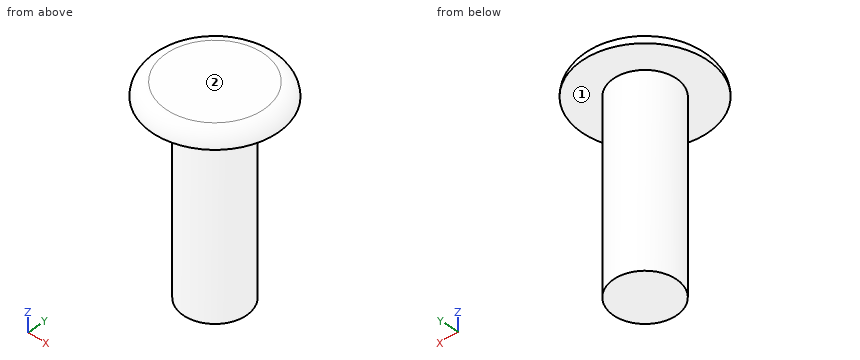
Autodesk Inventor part; units mm, degrees
ref_plane "YZ Plane" through (0, 0, 0) normal (1, 0, 0) x (0, 1, 0)
ref_plane "XZ Plane" through (0, 0, 0) normal (0, 1, 0) x (-1, 0, 0)
ref_plane "XY Plane" through (0, 0, 0) normal (0, 0, 1) x (1, 0, 0)
sketch "スケッチ1" plane through (0, 0, 0) normal (0, 0, 1) x (1, 0, 0)
  circle A0 centre (0, 0) radius 4
  dimension "d0" = 8
extrude "押し出し1" add sketch "スケッチ1" along normal blind 0.9
sketch "スケッチ2" plane through (0, 0, 0) normal (0, 0, -1) x (-1, 0, 0)
  circle A0 centre (0, 0) radius 2
  dimension "d3" = 4
extrude "押し出し2" add sketch "スケッチ2" along normal blind 12
thread "ねじ1"
fillet "フィレット1" radius 0.9 1 edges at (-4, 0, 0.9)
properties part number "ネジ低頭m4.12" material "鋼、高強度、低合金"
Model file for the job. Use its own axes, mm. Face numbers are marked on the shaded views. A direction names the side the tool comes from. Coordinates: 2 decimals unless noted, no trailing zeros. Loops run counter-clockwise (first coordinate to the right, second up) from the corner with the lowest first, then second, coordinate; pieces in that order, holes last. Notation, with made-up numbers: (-19.5, 22) -> (31.5, 22) arc R23 ccw to (31.5, 30) -> close; hole circle Ø3 at (1.5, -36.75). An arc over 180 degrees is marked (long way). Use one line per item in the form item = value. Start each with the question number.
(1) Cut at C-C on z = -3.25. Give the cut face in (x, y).
(2) Tool access for the marked faces 1 and 2: list every direction of +Z, -Z, +X, -X, +Y, -Y with a clear straight run to the whole face (end or side of a thin tool).
(3) Flat gauge pins, fed straight in: pin 1 (1 mm diameter, centred on x = 2.5, y = -1.5, fed in from -Z); pin 2 (4 mm diameter, centred on y = -0.5, z = -9, fed in from +X); pin 3 (3 mm diameter, centred on y = 2.5, z = -10.5, fed in from -X). Where does each tip first touch, or does it go through?
(4) Probe probe 1 along Z at (x, y) = (1, -2.25); probe 2 along Y at (x, z) = (-1.75, -2.25); probe 3 along X at (y, z) = (-1, -9.75). List the from-to ranges inside material, lowest first. Write a range as from..to.
Values:
q1.outline = circle Ø4 at (0, 0)
q2.face_1 = -Z
q2.face_2 = +Z, +X, -X, +Y, -Y
q3.pin_1 = 0
q3.pin_2 = 2
q3.pin_3 = -1.73
q4.probe_1 = 0..0.9
q4.probe_2 = -0.97..0.97
q4.probe_3 = -1.73..1.73
